Here's how the part is built. I have some questions about the finished solid (model axes, mm). A direction names the side the tool comes from. Give positions to 0.01 mm unless a question says otherwise; leave off trailing zeros. Loops run counter-clockwise (first coordinate to the right, second up) from the corner with the lowest first, then second, coordinate; pieces in that order, holes last.
Q1. Will these pins go through, and if not, where does the flat tip stop? P1, Ø4, axis at y = 16.5, z = -1.5, coming from the +X side; P2, Ø2, axis at x = -0.5, z = 3, coming from the -Y side; P3, Ø3, axis at x = -2, y = 24, coming from the +Z side.
Q2. If we section it at A-A (y = 10): Please give me the cut outline in (x, z).
Q3. I need wall thicknesses on line 1 (Z direction, x = -1.5, y = 8); line 2 (X direction, y = 25, z = -1); line 3 (Z direction, x = 0.5, y = 22). Which ranges of each line are inside material? Lowest first, please.
Q4. For faces 1 (the face through (2.2, 0, 0.1)), 2 (the face through (0, -2, 0)), which set-ups out of +Z, -Z, +X, -X, +Y, -Y let a thin tool reach every point of the face, with its end or its side?
Autodesk Inventor part; units mm, degrees
ref_plane "YZ Plane" through (0, 0, 0) normal (1, 0, 0) x (0, 1, 0)
ref_plane "XZ Plane" through (0, 0, 0) normal (0, 1, 0) x (-1, 0, 0)
ref_plane "XY Plane" through (0, 0, 0) normal (0, 0, 1) x (1, 0, 0)
sketch "Sketch1" plane through (0, 0, 0) normal (0, 1, 0) x (-1, 0, 0)
  circle A0 centre (0, 0) radius 1.85
  dimension "d0" = 3.7
extrude "Extrusion1" add sketch "Sketch1" along normal blind 30
sketch "Sketch2" plane through (0, 0, 0) normal (0, -1, 0) x (1, 0, 0)
  circle A0 centre (0, 0) radius 5
  dimension "d3" = 10
extrude "Extrusion2" add sketch "Sketch2" along normal blind 2
chamfer "Chamfer1" distance 1 angle 45 1 edges at (1.85, 30, 0)
fillet "Fillet1" radius 4.25 1 edges at (-5, -2, 0)
properties part number "Pin"
Check sheet entries:
1. P1: stops at x = 1.85
1. P2: stops at y = -1.95
1. P3: stops at z = 1.78
2. outline: circle Ø3.7 at (0, 0)
3. line 1: z = -1.08 to 1.08
3. line 2: x = -1.56 to 1.56
3. line 3: z = -1.78 to 1.78
4. face 1: +Y
4. face 2: +Z, -Z, +X, -X, -Y
